from build123d import *

# Parameters (mm, degrees)
SKETCH1_W           = 25.4
SKETCH1_H           = 25.4
BOSS_EXTRUDE1_DEPTH = 15.24
SKETCH2_W           = 12.7
SKETCH2_H           = 25.4
CUT_EXTRUDE1_DEPTH  = 10.16
SKETCH3_W           = 1.27
SKETCH3_H           = 10.16
CUT_EXTRUDE2_DEPTH  = 33.228986953
SKETCH4_W           = 25.4
SKETCH4_H           = 50.8
BOSS_EXTRUDE2_DEPTH = 2.54
SKETCH5_R           = 1.27
BOSS_EXTRUDE3_DEPTH = 7.62


with BuildPart() as part:
    # Sketch1 → Boss-Extrude1 (new body)
    with BuildSketch(Plane(origin=(0, 0, 0), x_dir=(1, 0, 0), z_dir=(0, 1, 0))):
        Rectangle(SKETCH1_W, SKETCH1_H)
    extrude(amount=BOSS_EXTRUDE1_DEPTH)

    # Sketch2 → Cut-Extrude1 (cut)
    with BuildSketch(Plane.XZ):
        Rectangle(SKETCH2_W, SKETCH2_H)
    extrude(amount=-CUT_EXTRUDE1_DEPTH, mode=Mode.SUBTRACT)

    # Sketch3 → Cut-Extrude2 (cut, through all)
    with BuildSketch(Plane.XY.offset(12.7)):
        with Locations((-12.065, 7.62)):
            Rectangle(SKETCH3_W, SKETCH3_H)
        with Locations((12.065, 7.62)):
            Rectangle(SKETCH3_W, SKETCH3_H)
    extrude(amount=-CUT_EXTRUDE2_DEPTH, mode=Mode.SUBTRACT)

    # Sketch4 → Boss-Extrude2 (add)
    with BuildSketch(Plane.XZ):
        with Locations((19.05, 0)):
            Rectangle(SKETCH4_W, SKETCH4_H)
    extrude(amount=BOSS_EXTRUDE2_DEPTH)

    # Sketch5 → Boss-Extrude3 (add)
    with BuildSketch(Plane.XZ.offset(2.54)):
        with Locations(Location((12.7, 19.05, 0), (0, 0, 90))):
            Circle(SKETCH5_R)
        with Locations(Location((22.098, 19.05, 0), (0, 0, 90))):
            Circle(SKETCH5_R)
        with Locations(Location((12.7, -19.05, 0), (0, 0, 90))):
            Circle(SKETCH5_R)
        with Locations(Location((22.098, -19.05, 0), (0, 0, 90))):
            Circle(SKETCH5_R)
    extrude(amount=BOSS_EXTRUDE3_DEPTH)


solid = part.part
Verification items for the finished model (mm, model axes). A direction names the side the tool comes from. Give positions to 0.01 mm unless a question says otherwise; leave off trailing zeros. Loops run counter-clockwise (first coordinate to the right, second up) from the corner with the lowest first, then second, coordinate; pieces in that order, holes last.
1) Sectioned sample at C-C, the plane y = 5.25. Enter the section's corners in (x, z).
2) Thickness scan on line 1 along X through (y, z) = (0.5, -2); line 2 along X through (y, z) = (3, -6); line 3 along X through (y, z) = (-1.75, -4). Record the ranges inside material, lowest first.
3) Set-up check for faces 4 (the flat face through (-10, 0, 0)), 5 (the flat face through (11.43, 8, 0)), 6 (the cylindrical face through (23.338, -6.297, 18.775)), 7 (the flat face through (6.35, 2, 0)): record each of +Z, -Z, +X, -X, +Y, -Y from which the full face is reachable in a straight line by a thin tool's end or side.
4) Sectioned sample at D-D, the plane z = -10. Enter the section's corners in (x, y), then the cut area to 3 significant figures.
5) Depth check by flat-ended pin: pin 1 Ø7.5 at (x, z) = (13, 1) entering from -Y; pin 2 Ø1.9 at (x, z) = (-11, 1) entering from -Y; pin 3 Ø6.5 at (x, z) = (0, -3.5) entering from -Y. Enter the tip coordinate at first touch or a pass-through.
6) Sectioned sample at A-A, the plane y = 0.75. Enter the section's corners in (x, z).
7) Draft check along Y on faces 1 (the flat face through (-12.7, 14, 0)), 2 (the flat face through (-12, 12.7, 0)), 3 (the flat face through (13, -10.16, 19)). Enter one of: pulls with the +Y half, pulls with the -Y half, needs draft (parallel to the pull), parting line crosses it, or undercut.
8) Sectioned sample at B-B, the plane z = -19.05. Enter the section's corners in (x, y), then the cut area to 3 significant figures.
Answers:
1. outline: (-11.43, -12.7) - (-6.35, -12.7) - (-6.35, 12.7) - (-11.43, 12.7) - close; (6.35, -12.7) - (11.43, -12.7) - (11.43, 12.7) - (6.35, 12.7) - close
2. line 1: x = -12.7 to -6.35, 6.35 to 12.7
2. line 2: x = -11.43 to -6.35, 6.35 to 11.43
2. line 3: x = 6.35 to 31.75
3. face 4: +Z, -Z, -X, -Y
3. face 5: +Z, -Z, +X
3. face 6: -Y
3. face 7: +Z, -Z, -Y
4. outline: (-12.7, 0) - (-6.35, 0) - (-6.35, 10.16) - (6.35, 10.16) - (6.35, -2.54) - (31.75, -2.54) - (31.75, 0) - (12.7, 0) - (12.7, 2.54) - (11.43, 2.54) - (11.43, 12.7) - (12.7, 12.7) - (12.7, 15.24) - (-12.7, 15.24) - (-12.7, 12.7) - (-11.43, 12.7) - (-11.43, 2.54) - (-12.7, 2.54) - close
4. area: 297 mm2
5. pin 1: stops at y = -2.54
5. pin 2: stops at y = 0
5. pin 3: stops at y = 10.16
6. outline: (-12.7, -12.7) - (-6.35, -12.7) - (-6.35, 12.7) - (-12.7, 12.7) - close; (6.35, -12.7) - (12.7, -12.7) - (12.7, 12.7) - (6.35, 12.7) - close
7. face 1: needs draft
7. face 2: undercut
7. face 3: pulls with the -Y half
8. outline: (6.35, -2.54) - (11.43, -2.54) - (11.43, -10.16) - (13.97, -10.16) - (13.97, -2.54) - (20.83, -2.54) - (20.83, -10.16) - (23.37, -10.16) - (23.37, -2.54) - (31.75, -2.54) - (31.75, 0) - (6.35, 0) - close
8. area: 103 mm2
